Input: dimensioned drawing with shaded views. Units: mm. Origin: part minimum x, y, z. Give positions to 0.01 mm unless a question says otherwise; leave off trailing zeros. Order: outer loops, then holes, each group sorted by start corner. A loop starts at its lowest first (then second) coordinate and runs counter-clockwise, first axis right, second up.
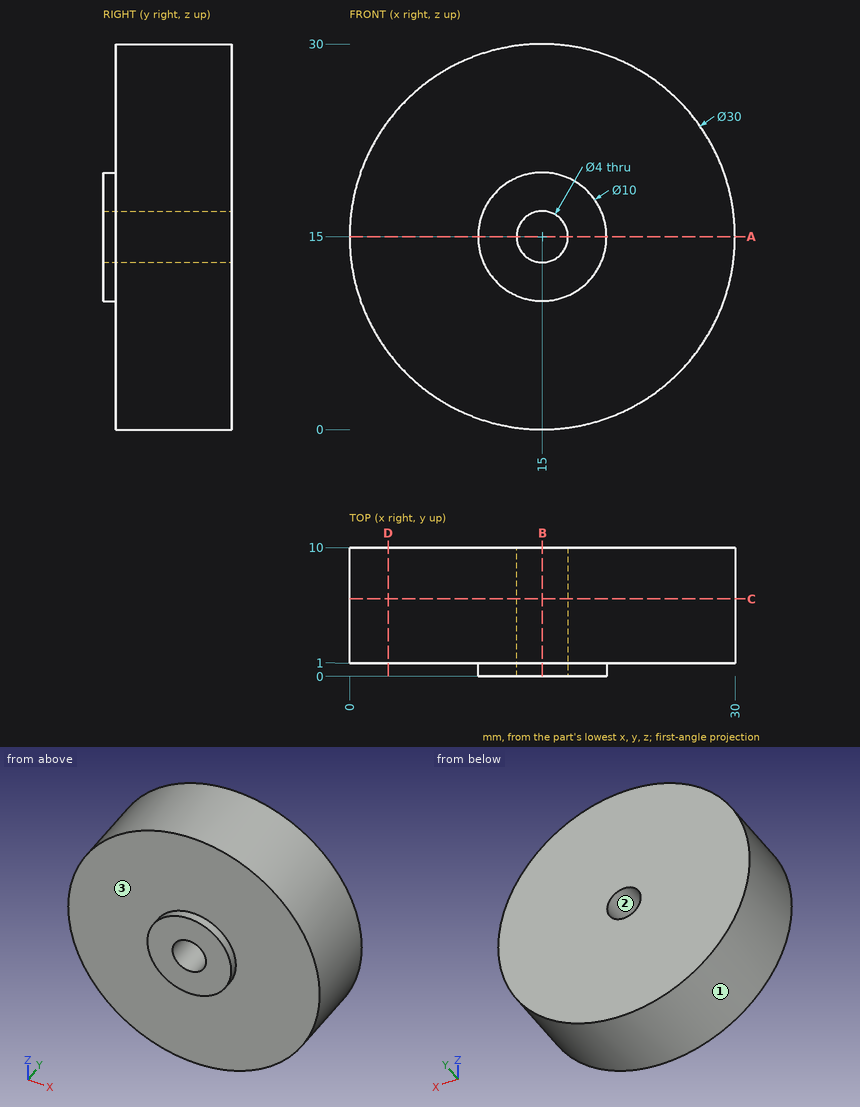
1) Cut plane B-B (x = 15). Return the cut outline in (y, z), then the cut area to 3 significant figures.
2) Cut plane C-C (y = 6). Return the cut outline in (x, z), then the cut area to 3 significant figures.
3) Pull-direction query (Z, two-part tool) for the marked faces 1, 2 and 3; classes: pulls with the +Z half, pulls with the -Z half, needs draft (parallel to the pull), parting line crosses it, or undercut.
4) Cut plane D-D (x = 3). Return the cut outline in (y, z), then the cut area to 3 significant figures.
5) Line query: probe 1 along Z at (x, y) = (15, 6.75); probe 2 along Y at (x, z) = (6.25, 18.5); probe 3 along Z at (x, y) = (16.75, 8). Output: solid intervals per line, ascending.
6) Cut plane A-A (z = 15). Return the cut outline in (x, y).
7) First-contact query: P1, Ø8, axis at x = 7, z = 6, coming from the -Y side; P2, Ø4, axis at y = 1, z = 7, coming from the -X side. Flat tips, straight axial feed; report the tip coordinate or a pass-through.
Geometry says:
1. outline: (0, 10) - (1, 10) - (1, 0) - (10, 0) - (10, 13) - (0, 13) - close; (0, 17) - (10, 17) - (10, 30) - (1, 30) - (1, 20) - (0, 20) - close
1. area: 240 mm2
2. outline: circle Ø30 at (15, 15); hole circle Ø4 at (15, 15)
2. area: 694 mm2
3. face 1: parting line crosses it
3. face 2: undercut
3. face 3: needs draft
4. outline: (1, 6) - (10, 6) - (10, 24) - (1, 24) - close
4. area: 162 mm2
5. probe 1: z = 0 to 13, 17 to 30
5. probe 2: y = 1 to 10
5. probe 3: z = 0.1 to 14.03, 15.97 to 29.9
6. outline: (0, 1) - (10, 1) - (10, 0) - (13, 0) - (13, 10) - (0, 10) - close; (17, 0) - (20, 0) - (20, 1) - (30, 1) - (30, 10) - (17, 10) - close
7. P1: stops at y = 1
7. P2: stops at x = 1.25
